For this review, take the finished solid that the model builds, in its own axes (mm). A direction names the side the tool comes from. Coordinates: 2 decimals unless noted, no trailing zeros. Write each loop counter-clockwise with the first axis right and the second up, starting at its lowest first coordinate (ties: lowest second). Pieces come first, ordered by that corner, then holes.
1) Insertion check: P1, Ø4, axis at x = -4, y = 22, coming from the -Z side; P2, Ø6, axis at x = 5.5, y = 28, coming from the -Z side; P3, Ø4, axis at y = 23, z = 0, coming from the -X side; P4, Ø3, axis at y = 21, z = -7, coming from the -X side. Each pin has a flat end and moves straight along its axis. Give the tip position at first contact, or say it passes through.
2) We need section C-C on y = 15. Write out the cut boundary in (x, z).
3) To check wall thickness, follow line 1 along Y through (x, z) = (-2.25, 7.75); line 2 along X through (y, z) = (5.5, 6.75); line 3 along Z through (x, y) = (-5, 11). State the ranges of each line that lie inside material, in increasing order.
4) We need section A-A on x = 0. Write out the cut boundary in (y, z).
5) For faces 1 (the face through (-5.4, 12, -0.1)), 2 (the face through (0, 6, 9)), list the 3-axis set-ups (+Z, -Z, +X, -X, +Y, -Y) from which the entire face can be reached by the end or side of a thin tool; tool diameter is ignored.
6) We need section B-B on z = 0. Write out the cut boundary in (x, y).
7) We need section D-D on z = 7.25. Write out the cut boundary in (x, y), then the cut area to 3 significant figures.
from build123d import *

# Parameters (mm, degrees)
EXTRUDE_1_DEPTH = 12
SKETCH_2_W      = 5
SKETCH_2_H      = 25


with BuildPart() as part:
    # 草图1 → 凸台-拉伸1 (new body)
    with BuildSketch(Plane(origin=(0, 12, 0), x_dir=(1, 0, 0), z_dir=(0, 1, 0))):
        with BuildLine():
            Line((-8, 4.123105626), (-8, -4.123105626))
            ThreePointArc((-8, -4.123105626), (0, -9), (8, -4.123105626))
            Line((8, -4.123105626), (8, 4.123105626))
            ThreePointArc((8, 4.123105626), (0, 9), (-8, 4.123105626))
        make_face()
    extrude(amount=-EXTRUDE_1_DEPTH)

    # 草图2 → 旋转1 (revolve)
    with BuildSketch(Plane.XY):
        with Locations((2.5, 24.5)):
            Rectangle(SKETCH_2_W, SKETCH_2_H)
    revolve(axis=Axis((0, 37, 0), (0, -1, 0)))


solid = part.part
Result:
1. P1: stops at z = -4.58
1. P2: stops at z = -4.33
1. P3: stops at x = -5
1. P4: passes through
2. outline: circle Ø10 at (0, 0)
3. line 1: y = 0 to 12
3. line 2: x = -5.95 to 5.95
3. line 3: z = -7.48 to 7.48
4. outline: (0, -9) - (12, -9) - (12, -5) - (37, -5) - (37, 5) - (12, 5) - (12, 9) - (0, 9) - close
5. face 1: +Y
5. face 2: +Z, +Y, -Y
6. outline: (-8, 0) - (8, 0) - (8, 12) - (5, 12) - (5, 37) - (-5, 37) - (-5, 12) - (-8, 12) - close
7. outline: (-5.33, 0) - (5.33, 0) - (5.33, 12) - (-5.33, 12) - close
7. area: 128 mm2
